Part model, mm, in its own coordinate system. A direction names the side the tool comes from. Coordinates: 2 decimals unless noted, no trailing zeros. Write each loop counter-clockwise with the first axis right and the second up, starting at its lowest first coordinate (ties: lowest second). Pieces come first, ordered by that corner, then holes. Notation, with made-up numbers: (-23.75, 66.25) - (31.25, 66.25) arc R28 cw to (31.25, 101.25) - close; hole circle Ø1 at (50, -11.5). An arc over 180 degrees is marked (long way). Use a Markdown table: item, result.
```python
from build123d import *

# Parameters (mm, degrees)
F0_W      = 60.8
F0_H      = 40.5
F1_DEPTH  = 1.5
F2_W      = 17.2
F2_H      = 7.7
F2_H_2    = 6.3
F3_DEPTH  = 10.8
F4_W      = 17.2
F4_H      = 9
F5_DEPTH  = 9.3
F6_W      = 10
F6_H      = 6
F6_W_2    = 9
F6_H_2    = 12.5
F7_DEPTH  = 2
F8_W      = 11
F8_H      = 5
F9_DEPTH  = 2
F10_W     = 25
F10_H     = 51
F10_W_2   = 11
F10_H_2   = 5
F11_DEPTH = 1.5
F12_W     = 8
F12_H     = 5.5
F12_W_2   = 7
F12_H_2   = 10.5
F13_DEPTH = 6
F14_W     = 20.5
F14_H     = 5
F15_DEPTH = 6.7
F17_D     = 3


with BuildPart() as f1:
    # F0 (on Top) → F1 (new body)
    with BuildSketch(Plane.XY):
        Rectangle(F0_W, F0_H)
    extrude(amount=F1_DEPTH)

    # F2 (on face) → F3 (join)
    with BuildSketch(Plane.XY.offset(1.5)):
        with Locations((16.4, -24.1)):
            Rectangle(F2_W, F2_H)
        with Locations((16.4, -17.1)):
            Rectangle(F2_W, F2_H_2)
    extrude(amount=F3_DEPTH)

    # F4 (on face) → F5 (join)
    with BuildSketch(Plane.XY.offset(1.5)):
        with Locations((-16.5, 13.75)):
            Rectangle(F4_W, F4_H)
    extrude(amount=F5_DEPTH)

    # F6 (on face) → F7 (join)
    with BuildSketch(Plane(origin=(0, 0, 0), x_dir=(1, 0, 0), z_dir=(0, 0, -1))):
        with Locations((-16.4, -13.25)):
            Rectangle(F6_W, F6_H)
        with Locations((1.9, 4.5)):
            Rectangle(F6_W_2, F6_H_2)
        with Locations((16.4, 15.25)):
            Rectangle(F6_W, F6_H)
    extrude(amount=F7_DEPTH)

    # F8 (on face) → F9 (join)
    with BuildSketch(Plane.XY.offset(10.8)):
        with Locations((-16.5, 13.75)):
            Rectangle(F8_W, F8_H)
    extrude(amount=F9_DEPTH)

    # F10 (on face) → F11 (join)
    with BuildSketch(Plane.XY.offset(12.8)):
        with Locations((-17.9, -5.25)):
            Rectangle(F10_W, F10_H)
        with Locations((-16.5, 13.75)):
            Rectangle(F10_W_2, F10_H_2, mode=Mode.SUBTRACT)
        with Locations((-16.5, 13.75)):
            Rectangle(F10_W_2, F10_H_2)
    extrude(amount=F11_DEPTH)

    # F12 (on face) → F13 (join)
    with BuildSketch(Plane.XY.offset(14.3)):
        with Locations((-34.4, 7.5)):
            Rectangle(F12_W, F12_H)
        with Locations((-26.9, 7.5)):
            Rectangle(F12_W_2, F12_H)
        with Locations((-26.9, -7)):
            Rectangle(F12_W_2, F12_H_2)
        with Locations((-34.4, -7)):
            Rectangle(F12_W, F12_H_2)
    extrude(amount=F13_DEPTH)

    # F14 (on face) → F15 (join)
    with BuildSketch(Plane.XY.offset(14.3)):
        with Locations((-19.15, -23.25)):
            Rectangle(F14_W, F14_H)
    extrude(amount=F15_DEPTH)

    # F17 (through all)
    with Locations(Plane.XY.offset(14.3)):
        with Locations((-7.9, -28.25), (-27.9, -28.25)):
            Hole(F17_D / 2)


solid = f1.part
```
Item 1: Band-saw the part on B-B, the plane z = 6.25. Give the cut face in (x, y), then the cut area to 3 significant figures.
From the geometry:
| item | result |
|---|---|
| outline | (-25.1, 9.25) - (-7.9, 9.25) - (-7.9, 18.25) - (-25.1, 18.25) - close; (7.8, -27.95) - (25, -27.95) - (25, -13.95) - (7.8, -13.95) - close |
| area | 396 mm^2 |
Item 2: Which spindle directions (+Z, -Z, +X, -X, +Y, -Y) get a long thin tool onto all of the face, cutting with end or side? Do faces 4 (the face through (-7.9, 14, 6)), 5 (the face through (-17, 16.25, 12)), 6 (the face through (16, -18.25, -1)), 7 (the face through (-17, 9.25, 6)). Say none if no direction does.
From the geometry:
| item | result |
|---|---|
| face 4 | +X, +Y, -Y |
| face 5 | +X, -X, +Y |
| face 6 | -Z, +X, -X, -Y |
| face 7 | +X, -X, -Y |
Item 3: Band-saw the part on A-A, the plane y = 7. Give the cut face in (x, z), then the cut area to 3 significant figures.
From the geometry:
| item | result |
|---|---|
| outline | (-38.4, 14.3) - (-30.4, 14.3) - (-30.4, 12.8) - (-5.4, 12.8) - (-5.4, 14.3) - (-23.4, 14.3) - (-23.4, 20.3) - (-38.4, 20.3) - close; (-30.4, 0) - (30.4, 0) - (30.4, 1.5) - (-30.4, 1.5) - close |
| area | 219 mm^2 |
Item 4: Two-plate mould, pull along Z, no slides. Class faces 1 (the face through (16, -24, 1.5)), 2 (the face through (-25.1, 14, 6)), 3 (the face through (7.8, -21, 7)): pulls with the +Z half, pulls with the -Z half, needs draft (parallel to the pull), parting line crosses it, or undercut.
From the geometry:
| item | result |
|---|---|
| face 1 | pulls with the -Z half |
| face 2 | undercut |
| face 3 | needs draft |
Item 5: Band-saw the part on C-C, the plane x = -27.9. Give the cut face in (y, z), then the cut area to 3 significant figures.
From the geometry:
| item | result |
|---|---|
| outline | (-30.75, 12.8) - (-29.75, 12.8) - (-29.75, 14.3) - (-30.75, 14.3) - close; (-26.75, 12.8) - (20.25, 12.8) - (20.25, 14.3) - (10.25, 14.3) - (10.25, 20.3) - (4.75, 20.3) - (4.75, 14.3) - (-1.75, 14.3) - (-1.75, 20.3) - (-12.25, 20.3) - (-12.25, 14.3) - (-20.75, 14.3) - (-20.75, 21) - (-25.75, 21) - (-25.75, 14.3) - (-26.75, 14.3) - close; (-20.25, 0) - (20.25, 0) - (20.25, 1.5) - (-20.25, 1.5) - close |
| area | 262 mm^2 |
Item 6: Drop flat-ended pins along their axis: P1, Ø2, axis at y = -23, z = 8.5, coming from the -X side; P2, Ø5, axis at y = -9, z = 5.5, coming from the +X side; P3, Ø2, axis at x = 0, z = -1.5, coming from the +Y side; P4, Ø15.5, axis at x = 15, y = -22, coming from the +Z side. Give the stop position or say it passes through.
From the geometry:
| item | result |
|---|---|
| P1 | x = 7.8 |
| P2 | through |
| P3 | y = 1.75 |
| P4 | z = 12.3 |
Item 7: Drill centre lines: probe 1 along Z at (x, y) = (-16, -1.5); probe 2 along Y at (x, z) = (-7.9, 13.1); probe 3 along Z at (x, y) = (-22.5, 17). Where is each one in solid material? Low to high.
From the geometry:
| item | result |
|---|---|
| probe 1 | 0 to 1.5, 12.8 to 14.3 |
| probe 2 | -30.75 to -29.75, -26.75 to 20.25 |
| probe 3 | 0 to 10.8, 12.8 to 14.3 |
Item 8: Band-saw the part on D-D, the plane z = 17.5. Give the cut face in (x, y).
From the geometry:
| item | result |
|---|---|
| outline | (-38.4, -12.25) - (-23.4, -12.25) - (-23.4, -1.75) - (-38.4, -1.75) - close; (-38.4, 4.75) - (-23.4, 4.75) - (-23.4, 10.25) - (-38.4, 10.25) - close; (-29.4, -25.75) - (-8.9, -25.75) - (-8.9, -20.75) - (-29.4, -20.75) - close |
